Autodesk Inventor part; units mm, degrees
ref_plane "YZ Plane" through (0, 0, 0) normal (1, 0, 0) x (0, 1, 0)
ref_plane "XZ Plane" through (0, 0, 0) normal (0, 1, 0) x (-1, 0, 0)
ref_plane "XY Plane" through (0, 0, 0) normal (0, 0, 1) x (1, 0, 0)
sketch "Sketch1" plane through (0, 0, 0) normal (0, 1, 0) x (-1, 0, 0)
  line L0 (0, 0) -> (139.7, 0)
  line L1 (139.7, 0) -> (139.7, -152.4)
  line L2 (139.7, -152.4) -> (0, -152.4)
  line L3 (0, -152.4) -> (0, 0)
  line L4 (139.7, -152.4) -> (127, -152.4)
  line L5 (114.3, -76.2) -> (114.3, -26.0366)
  line L6 (114.3, -26.0366) -> (139.7, -26.0366)
  line L7 (139.7, -26.0366) -> (139.7, -152.4)
  line L8 (127, -152.4) -> (76.2, -152.4)
  line L9 (76.2, -127) -> (76.2, -76.2)
  line L10 (76.2, -76.2) -> (114.3, -76.2)
  line L11 (76.2, -152.4) -> (50.8, -152.4)
  line L12 (50.8, -152.4) -> (50.8, -127)
  line L13 (50.8, -127) -> (76.2, -127)
  circle A0 centre (12.7, -12.7) radius 6.35 construction
  circle A1 centre (12.7, -31.75) radius 6.35 construction
  circle A2 centre (12.7, -50.8) radius 6.35 construction
  circle A3 centre (12.7, -69.85) radius 6.35 construction
  circle A4 centre (12.7, -88.9) radius 6.35 construction
  circle A5 centre (12.7, -107.95) radius 6.35 construction
  circle A6 centre (12.7, -127) radius 6.35 construction
  circle A7 centre (31.75, -12.7) radius 6.35 construction
  circle A8 centre (31.75, -31.75) radius 6.35 construction
  circle A9 centre (31.75, -50.8) radius 6.35 construction
  circle A10 centre (31.75, -69.85) radius 6.35 construction
  circle A11 centre (31.75, -88.9) radius 6.35 construction
  circle A12 centre (31.75, -107.95) radius 6.35 construction
  circle A13 centre (31.75, -127) radius 6.35 construction
  circle A14 centre (12.7, -12.7) radius 6.223
  circle A15 centre (12.7, -31.75) radius 6.2357
  circle A16 centre (12.7, -50.8) radius 6.2484
  circle A17 centre (12.7, -69.85) radius 6.2611
  circle A18 centre (12.7, -88.9) radius 6.2738
  circle A19 centre (12.7, -107.95) radius 6.2865
  circle A20 centre (12.7, -127) radius 6.2992
  circle A21 centre (31.75, -12.7) radius 6.3119
  circle A22 centre (31.75, -31.75) radius 6.3246
  circle A23 centre (31.75, -50.8) radius 6.3373
  circle A24 centre (31.75, -69.85) radius 6.35
  circle A25 centre (31.75, -88.9) radius 6.3627
  circle A26 centre (31.75, -107.95) radius 6.3754
  circle A27 centre (31.75, -127) radius 6.3881
  circle A28 centre (50.8, -12.7) radius 6.4008
  circle A29 centre (50.8, -31.75) radius 6.4135
  circle A30 centre (50.8, -50.8) radius 6.4262
  circle A31 centre (50.8, -69.85) radius 6.4389
  circle A32 centre (50.8, -88.9) radius 6.4516
  circle A33 centre (50.8, -107.95) radius 6.4643
  circle A34 centre (76.2, -12.7) radius 6.35
  circle A35 centre (76.2, -31.75) radius 6.35
  circle A36 centre (76.2, -50.8) radius 6.35
  line L14 (6.4177, -6.5588) -> (6.4177, -14.6901) construction
  line L15 (8.0052, -4.9713) -> (8.0052, -13.1026) construction
  circle A37 centre (133.35, -6.35) radius 1.778
  circle A38 centre (133.35, -12.7) radius 1.7907
  circle A39 centre (133.35, -19.05) radius 1.8034
  circle A40 centre (127, -6.35) radius 1.8161
  circle A41 centre (127, -12.7) radius 1.8288
  circle A42 centre (127, -19.05) radius 1.8415
  circle A43 centre (120.65, -6.35) radius 1.8542
  circle A44 centre (120.65, -12.7) radius 1.8669
  circle A45 centre (120.65, -19.05) radius 1.8796
  circle A46 centre (114.3, -6.35) radius 1.8923
  circle A47 centre (114.3, -12.7) radius 1.8669
  circle A48 centre (114.3, -19.05) radius 1.8796
  circle A49 centre (107.95, -6.35) radius 1.8923
  circle A50 centre (107.95, -12.7) radius 1.8669
  circle A51 centre (107.95, -19.05) radius 1.8796
  circle A52 centre (107.95, -25.4) radius 1.8923
  circle A53 centre (107.95, -31.75) radius 1.905
  circle A54 centre (107.95, -38.1) radius 1.9177
  circle A55 centre (107.95, -44.45) radius 1.9304
  circle A56 centre (107.95, -50.8) radius 1.9431
  circle A57 centre (107.95, -57.15) radius 1.9558
  circle A58 centre (107.95, -63.5) radius 1.9685
  dimension "d0" = 139.7
  dimension "d1" = 152.4
  dimension "d3" = 127
  dimension "d5" = 76.2
  dimension "d7" = 25.4
  dimension "d8" = 12.7
  dimension "d9" = 12.7
  dimension "d10" = 12.7
  dimension "d13" = 19.05
  dimension "d16" = 19.05
  dimension "d19" = 12.446
  dimension "d20" = 12.4714
  dimension "d21" = 12.4968
  dimension "d22" = 12.5222
  dimension "d23" = 12.5476
  dimension "d24" = 12.573
  dimension "d25" = 12.5984
  dimension "d26" = 12.6238
  dimension "d27" = 12.6492
  dimension "d28" = 12.6746
  dimension "d29" = 12.7
  dimension "d30" = 12.7254
  dimension "d31" = 12.7508
  dimension "d32" = 12.7762
  dimension "d33" = 12.8016
  dimension "d34" = 12.827
  dimension "d35" = 12.8524
  dimension "d36" = 12.8778
  dimension "d37" = 12.9032
  dimension "d38" = 12.9286
  dimension "d39" = 12.7
  dimension "d40" = 12.7
  dimension "d41" = 12.7
  dimension "d44" = 50.8
  dimension "d45" = 25.4
  dimension "d46" = 25.4
  dimension "d47" = 3.556
  dimension "d48" = 6.35
  dimension "d49" = 6.35
  dimension "d50" = 3.5814
  dimension "d51" = 6.35
  dimension "d52" = 3.6068
  dimension "d53" = 6.35
  dimension "d54" = 3.6322
  dimension "d55" = 6.35
  dimension "d56" = 3.6576
  dimension "d57" = 3.683
  dimension "d58" = 3.7084
  dimension "d59" = 6.35
  dimension "d60" = 3.7338
  dimension "d61" = 3.7592
  dimension "d62" = 3.7846
  dimension "d63" = 6.35
  dimension "d64" = 3.7338
  dimension "d65" = 3.7592
  dimension "d66" = 3.7846
  dimension "d67" = 6.35
  dimension "d68" = 3.7338
  dimension "d69" = 3.7592
  dimension "d70" = 3.7846
  dimension "d71" = 6.35
  dimension "d72" = 3.81
  dimension "d73" = 3.8354
  dimension "d74" = 3.8608
extrude "Extrusion1" add sketch "Sketch1" along normal blind 6.35 contours L0 L1 L6 L5 L10 L9 L13 L12 L2 L3
sketch "Sketch2" plane through (0, 6.35, 0) normal (0, 1, 0) x (1, 0, 0)
  line L0 (-4.5975, 9.3875) -> (-4.5975, 17.5188) construction
  line L1 (-4.5975, 17.5188) -> (-1.4235, 17.5188) construction
  line L2 (-1.4235, 17.5188) -> (-1.4235, 9.3875) construction
  line L3 (-1.4235, 9.3875) -> (-4.5975, 9.3875) construction
  point P0 (0, 0)
sketch "Sketch3" plane through (0, 6.35, 0) normal (0, 1, 0) x (1, 0, 0)
  point P0 (0, 0)
sketch "Sketch4" plane through (0, 6.35, 0) normal (0, 1, 0) x (1, 0, 0)
  line L0 (-95.25, 12.7) -> (-95.2246, 12.7)
  line L1 (-95.2246, 12.7) -> (-95.2246, 38.1)
  line L2 (-95.2246, 38.1) -> (-95.25, 38.1)
  line L3 (-95.25, 38.1) -> (-95.25, 12.7)
  line L4 (-139.7, 26.0366) -> (-139.7, 0)
  line L5 (-139.7, 0) -> (0, 0)
  dimension "d84" = 0.0254
  dimension "d85" = 25.4
  dimension "d86" = 44.45
  dimension "d87" = 12.7
extrude "Extrusion2" cut sketch "Sketch4" against normal through all
properties part number "Test laser cutter tolerances"
Can you work these out from the model? Positions are in its coordinate system, mm. A direction names the side the tool comes from. Round coordinates to 2 decimals unless told otherwise and drop trailing zeros. Order: outer loops, then holes, each group sorted by start corner. A loop starts at its lowest first (then second) coordinate and runs counter-clockwise, first axis right, second up.
(1) If we section it at B-B (x = -133.35): Please give me the cut outline in (y, z).
Results are:
outline: (0, -26.04) - (6.35, -26.04) - (6.35, -20.85) - (0, -20.85) - close; (0, -17.25) - (6.35, -17.25) - (6.35, -14.49) - (0, -14.49) - close; (0, -10.91) - (6.35, -10.91) - (6.35, -8.13) - (0, -8.13) - close; (0, -4.57) - (6.35, -4.57) - (6.35, 0) - (0, 0) - close
(2) We'd pull the mould along Z, two halves only. Please class faces 1 (the face through (-26, 3, -152.4)), 2 (the face through (-109.8, 3.1, -51.4)), 3 (the face through (-53, 6.35, -58)): +Z half, -Z half, draft (parallel to the pull), parting line (faces both ways), or undercut.
Results are:
face 1: -Z half
face 2: undercut
face 3: draft
(3) If we section it at A-A (x = -12.7): Count the separate pieces of the cut face and the enclosed holes in it, plus the area to 3 significant figures.
Results are:
separate pieces: 8
enclosed holes: 0
area: 411 mm2
(4) If I drill on L1, parallel to Z at x = -76.5, y = 5.5; L2, parallel to Z at x = -75, y = 5.5; L3, parallel to X at y = 0.5, z = -66, over which ranges is the centre line in solid material (lowest first)?
Results are:
L1: z = -76.2 to -57.14, -44.46 to -38.09, -25.41 to -19.04, -6.36 to 0
L2: z = -127 to -57.04, -44.56 to -37.99, -25.51 to -18.94, -6.46 to 0
L3: x = -114.3 to -55.96, -45.64 to -36.8, -26.7 to -17.64, -7.76 to 0
(5) On a 3-axis mill with a long thin cutter (end or side, diameter ignored), from which of +Z, -Z, +X, -X, +Y, -Y can I reach the whole of each face in a straight line? I mean faces 4 (the face through (-131.55, 3.13, -19.13)), 5 (the face through (-76.2, 3, -102)). Say none if no direction works.
Results are:
face 4: +Y, -Y
face 5: -Z, -X, +Y, -Y
(6) If we section it at C-C (z = -69.85): Please give me the cut outline in (x, y), plus the area to 3 significant figures.
Results are:
outline: (-114.3, 0) - (-57.24, 0) - (-57.24, 6.35) - (-114.3, 6.35) - close; (-44.36, 0) - (-38.1, 0) - (-38.1, 6.35) - (-44.36, 6.35) - close; (-25.4, 0) - (-18.96, 0) - (-18.96, 6.35) - (-25.4, 6.35) - close; (-6.44, 0) - (0, 0) - (0, 6.35) - (-6.44, 6.35) - close
area: 484 mm2
(7) I'm going to push a flat-ended pin straight in: pin 1 (1 mm diameter, centred on x = -63.5, y = 1, fed in from -Z). Where does the tip first touch, or does it pass through?
Results are:
pin 1: stops at z = -127
(8) If we section it at D-D (z = -50.8): Please give me the cut outline in (x, y), plus the area to 3 significant figures.
Results are:
outline: (-114.3, 0) - (-109.89, 0) - (-109.89, 6.35) - (-114.3, 6.35) - close; (-106.01, 0) - (-82.55, 0) - (-82.55, 6.35) - (-106.01, 6.35) - close; (-69.85, 0) - (-57.23, 0) - (-57.23, 6.35) - (-69.85, 6.35) - close; (-44.37, 0) - (-38.09, 0) - (-38.09, 6.35) - (-44.37, 6.35) - close; (-25.41, 0) - (-18.95, 0) - (-18.95, 6.35) - (-25.41, 6.35) - close; (-6.45, 0) - (0, 0) - (0, 6.35) - (-6.45, 6.35) - close
area: 379 mm2
